For this review, take the finished solid that the model builds, in its own axes (mm). A direction names the side the tool comes from. Give positions to 0.01 mm unless a question says otherwise; leave off trailing zeros. Order: outer loops, then holes, each group sorted by start corner. A loop starts at its lowest first (then second) coordinate and runs counter-clockwise, first axis right, second up.
Item 1: Consider section B-B (z = 52). Give the boundary of the cut face in (x, y).
Item 2: Consider section C-C (x = 321). Give the boundary of the cut face in (y, z), plus the area to 3 significant figures.
Item 3: Consider section A-A (y = -60). Give the boundary of the cut face in (x, z), plus the area to 3 significant figures.
Item 4: The part is to be moulded in two halves that separate along X. For faces 1 (the flat face through (257, 0, 45)), 2 (the flat face through (494.3, -26.47, 45.36)), 3 (the flat face through (26.47, -25.7, 45.36)), 4 (the flat face through (520, -69, 45)), say which applies: released by +X, released by -X, zero draft, split by the parting line, or undercut.
Item 5: Consider section D-D (y = -101). Give the boundary of the cut face in (x, z), plus the area to 3 significant figures.
Item 6: For probe 1 along X at (y, z) = (-71, 34.5); probe 2 along X at (y, z) = (-119, 68); probe 3 along Y at (x, z) = (79.5, 8.5), list the stretches that pass through material, from the lowest coordinate up.
Item 7: For P1, Ø3, axis at x = 379.5, z = 16, coming from the -Y side; P2, Ø1, axis at x = 521, z = 30, coming from the -Y side; P3, Ø10, axis at y = -27, z = 59, coming from the -X side, all flat-tipped, find the tip position at first contact; note any pin that passes through.
Item 8: Machinability: for faces 5 (the flat face through (-2, -109, 45)), 6 (the flat face through (0, -111, 45)), which of the approach directions +Z, -Z, +X, -X, +Y, -Y give a long, thin tool a straight path to every point of the face, cutting with its end or side? Answer none if there is none.
```python
from build123d import *

# Parameters (mm, degrees)
EXTRU_MINCE1_DEPTH        = 92
CONVERTIR_VOLUME1_DEPTH   = 92
CONVERTIR_VOLUME1_2_DEPTH = 92


# Read off the part's stored shape, not the designer's step: Convertir-Volume1
with BuildPart() as part:
    # Esquisse1 → Extru.-Mince1 (new body)
    with BuildSketch(Plane.XY):
        Polygon((520, -82), (520, -55), (465, 0), (55, 0), (0, -55), (0, -165), (10, -165), (10, -59.142135624), (59.142135624, -10), (460.857864376, -10), (510, -59.142135624), (510, -82), align=None)
    extrude(amount=EXTRU_MINCE1_DEPTH)

    # Convertir-Volume1 outline → Convertir-Volume1 (cut)
    with BuildSketch(Plane.XY):
        with BuildLine():
            Line((0, -55.414213562), (0, -165))
            Line((0, -165), (10, -165))
            Line((10, -165), (10, -59.142135624))
            Line((10, -59.142135624), (59.142135624, -10))
            Line((59.142135624, -10), (460.857864376, -10))
            Line((460.857864376, -10), (510, -59.142135624))
            Line((510, -59.142135624), (510, -82))
            Line((510, -82), (520, -82))
            Line((520, -82), (520, -55.414213562))
            ThreePointArc((520, -55.414213562), (519.923879533, -55.03153013), (519.707106781, -54.707106781))
            Line((519.707106781, -54.707106781), (465.292893219, -0.292893219))
            ThreePointArc((465.292893219, -0.292893219), (464.96846987, -0.076120467), (464.585786438, 0))
            Line((464.585786438, 0), (55.414213562, 0))
            ThreePointArc((55.414213562, 0), (55.03153013, -0.076120467), (54.707106781, -0.292893219))
            Line((54.707106781, -0.292893219), (0.292893219, -54.707106781))
            ThreePointArc((0.292893219, -54.707106781), (0.076120467, -55.03153013), (0, -55.414213562))
        make_face()
    extrude(amount=CONVERTIR_VOLUME1_DEPTH, mode=Mode.SUBTRACT)

    # Convertir-Volume1 2 outline → Convertir-Volume1 2 (add)
    with BuildSketch(Plane.XY):
        with BuildLine():
            Line((-2, -55.414213562), (-2, -165))
            Line((-2, -165), (0, -165))
            Line((0, -165), (0, -55))
            Line((0, -55), (55, 0))
            Line((55, 0), (465, 0))
            Line((465, 0), (520, -55))
            Line((520, -55), (520, -82))
            Line((520, -82), (522, -82))
            Line((522, -82), (522, -55.414213562))
            ThreePointArc((522, -55.414213562), (521.771638598, -54.266163265), (521.121320344, -53.292893219))
            Line((521.121320344, -53.292893219), (466.707106781, 1.121320344))
            ThreePointArc((466.707106781, 1.121320344), (465.733836735, 1.771638598), (464.585786438, 2))
            Line((464.585786438, 2), (55.414213562, 2))
            ThreePointArc((55.414213562, 2), (54.266163265, 1.771638598), (53.292893219, 1.121320344))
            Line((53.292893219, 1.121320344), (-1.121320344, -53.292893219))
            ThreePointArc((-1.121320344, -53.292893219), (-1.771638598, -54.266163265), (-2, -55.414213562))
        make_face()
    extrude(amount=CONVERTIR_VOLUME1_2_DEPTH)


solid = part.part
```
Resolved:
1. outline: (-2, -165) - (0, -165) - (0, -55.41) arc R1 cw to (0.29, -54.71) - (54.71, -0.29) arc R1 cw to (55.41, 0) - (464.59, 0) arc R1 cw to (465.29, -0.29) - (519.71, -54.71) arc R1 cw to (520, -55.41) - (520, -82) - (522, -82) - (522, -55.41) arc R3 ccw to (521.12, -53.29) - (466.71, 1.12) arc R3 ccw to (464.59, 2) - (55.41, 2) arc R3 ccw to (53.29, 1.12) - (-1.12, -53.29) arc R3 ccw to (-2, -55.41) - close
2. outline: (0, 0) - (2, 0) - (2, 92) - (0, 92) - close
2. area: 184 mm2
3. outline: (-2, 0) - (0, 0) - (0, 92) - (-2, 92) - close; (520, 0) - (522, 0) - (522, 92) - (520, 92) - close
3. area: 368 mm2
4. face 1: undercut
4. face 2: released by +X
4. face 3: released by -X
4. face 4: undercut
5. outline: (-2, 0) - (0, 0) - (0, 92) - (-2, 92) - close
5. area: 184 mm2
6. probe 1: x = -2 to 0, 520 to 522
6. probe 2: x = -2 to 0
6. probe 3: y = 0 to 2
7. P1: stops at y = 0
7. P2: stops at y = -82
7. P3: stops at x = 20.17
8. face 5: +Z, -Z, -X, +Y, -Y
8. face 6: +Z, -Z, -Y
